Source: CAD feature listing. Evaluate the final solid. Frame: model axes, mm. A direction names the side the tool comes from. Coordinates: 2 decimals unless noted, no trailing zeros. Order: outer loops, then holes, each group sorted by start corner. A loop starts at its lowest first (then second) coordinate and runs counter-clockwise, first axis right, second up.
```python
from build123d import *

# Parameters (mm, degrees)
SKETCH1_R           = 2.7
BOSS_EXTRUDE1_DEPTH = 6.35


with BuildPart() as part:
    # Sketch1 → Boss-Extrude1 (new body)
    with BuildSketch(Plane(origin=(0, 0, 0), x_dir=(0, 0, -1), z_dir=(1, 0, 0))):
        with BuildLine():
            Line((-44.45, 57.15), (-44.45, 50.8))
            Line((-44.45, 50.8), (-55.5, 50.8))
            Line((-55.5, 50.8), (-55.5, 45.8))
            Line((-55.5, 45.8), (-54.3, 45.8))
            Line((-54.3, 45.8), (-54.3, 43.3))
            Line((-54.3, 43.3), (-55.5, 43.3))
            Line((-55.5, 43.3), (-55.5, 40.8))
            Line((-55.5, 40.8), (-58.8, 40.8))
            Line((-58.8, 40.8), (-58.8, 43.3))
            Line((-58.8, 43.3), (-60, 43.3))
            Line((-60, 43.3), (-60, 45.8))
            Line((-60, 45.8), (-58.8, 45.8))
            Line((-58.8, 45.8), (-58.8, 50.8))
            Line((-58.8, 50.8), (-69.85, 50.8))
            Line((-69.85, 50.8), (-69.85, 57.15))
            Line((-69.85, 57.15), (-152.4, 57.15))
            Line((-152.4, 57.15), (-152.4, 50.8))
            Line((-152.4, 50.8), (-163.45, 50.8))
            Line((-163.45, 50.8), (-163.45, 45.8))
            Line((-163.45, 45.8), (-162.25, 45.8))
            Line((-162.25, 45.8), (-162.25, 43.3))
            Line((-162.25, 43.3), (-163.45, 43.3))
            Line((-163.45, 43.3), (-163.45, 40.8))
            Line((-163.45, 40.8), (-166.75, 40.8))
            Line((-166.75, 40.8), (-166.75, 43.3))
            Line((-166.75, 43.3), (-167.95, 43.3))
            Line((-167.95, 43.3), (-167.95, 45.8))
            Line((-167.95, 45.8), (-166.75, 45.8))
            Line((-166.75, 45.8), (-166.75, 50.8))
            Line((-166.75, 50.8), (-177.8, 50.8))
            Line((-177.8, 50.8), (-177.8, 57.15))
            Line((-177.8, 57.15), (-215.9, 57.15))
            Line((-215.9, 57.15), (-215.9, 47.6875))
            Line((-215.9, 47.6875), (-210.9, 47.6875))
            Line((-210.9, 47.6875), (-210.9, 48.8875))
            Line((-210.9, 48.8875), (-208.4, 48.8875))
            Line((-208.4, 48.8875), (-208.4, 47.6875))
            Line((-208.4, 47.6875), (-205.9, 47.6875))
            Line((-205.9, 47.6875), (-205.9, 44.3875))
            Line((-205.9, 44.3875), (-208.4, 44.3875))
            Line((-208.4, 44.3875), (-208.4, 43.1875))
            Line((-208.4, 43.1875), (-210.9, 43.1875))
            Line((-210.9, 43.1875), (-210.9, 44.3875))
            Line((-210.9, 44.3875), (-215.9, 44.3875))
            Line((-215.9, 44.3875), (-215.9, 34.925))
            Line((-215.9, 34.925), (-222.25, 34.925))
            Line((-222.25, 34.925), (-222.25, 22.225))
            Line((-222.25, 22.225), (-215.9, 22.225))
            Line((-215.9, 22.225), (-215.9, 12.7625))
            Line((-215.9, 12.7625), (-210.9, 12.7625))
            Line((-210.9, 12.7625), (-210.9, 13.9625))
            Line((-210.9, 13.9625), (-208.4, 13.9625))
            Line((-208.4, 13.9625), (-208.4, 12.7625))
            Line((-208.4, 12.7625), (-205.9, 12.7625))
            Line((-205.9, 12.7625), (-205.9, 9.4625))
            Line((-205.9, 9.4625), (-208.4, 9.4625))
            Line((-208.4, 9.4625), (-208.4, 8.2625))
            Line((-208.4, 8.2625), (-210.9, 8.2625))
            Line((-210.9, 8.2625), (-210.9, 9.4625))
            Line((-210.9, 9.4625), (-215.9, 9.4625))
            Line((-215.9, 9.4625), (-215.9, 0))
            Line((-215.9, 0), (-160.59896879, 0))
            ThreePointArc((-160.59896879, 0), (-158.861506462, 0.306361486), (-157.333607733, 1.188494229))
            Line((-157.333607733, 1.188494229), (-139.588074729, 16.078764428))
            ThreePointArc((-139.588074729, 16.078764428), (-135.768327906, 18.284096284), (-131.424672086, 19.05))
            Line((-131.424672086, 19.05), (131.424672086, 19.05))
            ThreePointArc((131.424672086, 19.05), (135.768327906, 18.284096284), (139.588074729, 16.078764428))
            Line((139.588074729, 16.078764428), (157.333607733, 1.188494229))
            ThreePointArc((157.333607733, 1.188494229), (158.861506462, 0.306361486), (160.59896879, 0))
            Line((160.59896879, 0), (215.9, 0))
            Line((215.9, 0), (215.9, 9.4625))
            Line((215.9, 9.4625), (210.9, 9.4625))
            Line((210.9, 9.4625), (210.9, 8.2625))
            Line((210.9, 8.2625), (208.4, 8.2625))
            Line((208.4, 8.2625), (208.4, 9.4625))
            Line((208.4, 9.4625), (205.9, 9.4625))
            Line((205.9, 9.4625), (205.9, 12.7625))
            Line((205.9, 12.7625), (208.4, 12.7625))
            Line((208.4, 12.7625), (208.4, 13.9625))
            Line((208.4, 13.9625), (210.9, 13.9625))
            Line((210.9, 13.9625), (210.9, 12.7625))
            Line((210.9, 12.7625), (215.9, 12.7625))
            Line((215.9, 12.7625), (215.9, 22.225))
            Line((215.9, 22.225), (222.25, 22.225))
            Line((222.25, 22.225), (222.25, 34.925))
            Line((222.25, 34.925), (215.9, 34.925))
            Line((215.9, 34.925), (215.9, 44.3875))
            Line((215.9, 44.3875), (210.9, 44.3875))
            Line((210.9, 44.3875), (210.9, 43.1875))
            Line((210.9, 43.1875), (208.4, 43.1875))
            Line((208.4, 43.1875), (208.4, 44.3875))
            Line((208.4, 44.3875), (205.9, 44.3875))
            Line((205.9, 44.3875), (205.9, 47.6875))
            Line((205.9, 47.6875), (208.4, 47.6875))
            Line((208.4, 47.6875), (208.4, 48.8875))
            Line((208.4, 48.8875), (210.9, 48.8875))
            Line((210.9, 48.8875), (210.9, 47.6875))
            Line((210.9, 47.6875), (215.9, 47.6875))
            Line((215.9, 47.6875), (215.9, 57.15))
            Line((215.9, 57.15), (177.8, 57.15))
            Line((177.8, 57.15), (177.8, 50.8))
            Line((177.8, 50.8), (163.575, 50.8))
            Line((163.575, 50.8), (163.575, 45.8))
            Line((163.575, 45.8), (164.775, 45.8))
            Line((164.775, 45.8), (164.775, 43.3))
            Line((164.775, 43.3), (163.575, 43.3))
            Line((163.575, 43.3), (163.575, 40.8))
            Line((163.575, 40.8), (160.275, 40.8))
            Line((160.275, 40.8), (160.275, 43.3))
            Line((160.275, 43.3), (159.075, 43.3))
            Line((159.075, 43.3), (159.075, 45.8))
            Line((159.075, 45.8), (160.275, 45.8))
            Line((160.275, 45.8), (160.275, 50.8))
            Line((160.275, 50.8), (146.05, 50.8))
            Line((146.05, 50.8), (146.05, 57.15))
            Line((146.05, 57.15), (63.5, 57.15))
            Line((63.5, 57.15), (63.5, 50.8))
            Line((63.5, 50.8), (52.45, 50.8))
            Line((52.45, 50.8), (52.45, 45.8))
            Line((52.45, 45.8), (53.65, 45.8))
            Line((53.65, 45.8), (53.65, 43.3))
            Line((53.65, 43.3), (52.45, 43.3))
            Line((52.45, 43.3), (52.45, 40.8))
            Line((52.45, 40.8), (49.15, 40.8))
            Line((49.15, 40.8), (49.15, 43.3))
            Line((49.15, 43.3), (47.95, 43.3))
            Line((47.95, 43.3), (47.95, 45.8))
            Line((47.95, 45.8), (49.15, 45.8))
            Line((49.15, 45.8), (49.15, 50.8))
            Line((49.15, 50.8), (38.1, 50.8))
            Line((38.1, 50.8), (38.1, 57.15))
            Line((38.1, 57.15), (-44.45, 57.15))
        make_face()
        with Locations((105.388301448, 33.74898)):
            Circle(SKETCH1_R, mode=Mode.SUBTRACT)
        with Locations((29.188301448, 33.74898)):
            Circle(SKETCH1_R, mode=Mode.SUBTRACT)
        with Locations((181.588301448, 33.74898)):
            Circle(SKETCH1_R, mode=Mode.SUBTRACT)
    extrude(amount=-BOSS_EXTRUDE1_DEPTH)


solid = part.part
```
1. Section query A-A, the plane z = -74.5. Output: boundary loops of the cut face in (x, y).
2. Draft query along Z for faces 3 (the flat face through (-6.35, 35, 3)), 4 (the flat face through (-3.131, 8.738, -148.337)). Return one class per face: +Z half, -Z half, draft (parallel to the pull), parting line (faces both ways), or undercut.
3. Material intervals for line 1 along Z through (x, y) = (-1, 41.5) (3 decimals); line 2 along Z through (x, y) = (-4.5, 34); line 3 along Z through (x, y) = (-3.75, 54), sorted ascending.
4. Contact query for flat-ended pins moving along their axis: P1, Ø1.6, axis at x = -3, y = 10.5, coming from the -Z side; P2, Ø0.6, axis at x = -2.5, y = 8.5, coming from the +Z side; P3, Ø1.5, axis at x = -2, z = 21, coming from the -Y side. Output: stop coordinate, or through.
5. Access query for faces 1 (the flat face through (0, 35, 3)), 2 (the flat face through (-3.131, 8.529, 148.585)). Directions: +Z, -Z, +X, -X, +Y, -Y. A direction counts if a zero-diameter tool reaches every point of the face in a straight line with its end or side. Return the directions, or none.
6. Section query B-B, the plane x = -2.5. Count the separate pieces of the cut face and the enclosed holes in it, plus the area to 3 significant figures.
Answer key:
1. outline: (-6.35, 19.05) - (0, 19.05) - (0, 57.15) - (-6.35, 57.15) - close
2. face 3: draft
2. face 4: undercut
3. line 1: z = -215.9 to -163.575, -160.275 to -52.45, -49.15 to 55.5, 58.8 to 163.45, 166.75 to 215.9
3. line 2: z = -222.25 to -184.28, -178.9 to -108.08, -102.7 to -31.88, -26.5 to 222.25
3. line 3: z = -215.9 to -177.8, -146.05 to -63.5, -38.1 to 44.45, 69.85 to 152.4, 177.8 to 215.9
4. P1: stops at z = -205.9
4. P2: stops at z = 215.9
4. P3: stops at y = 19.05
5. face 1: +Z, -Z, +X, +Y, -Y
5. face 2: +X, -X, -Y
6. separate pieces: 1
6. enclosed holes: 3
6. area: 18,200 mm2
